```python
from build123d import *

# Parameters (mm, degrees)
BOSS_EXTRUDE1_DEPTH = 11.1125
SKETCH2_R           = 3.5687
CUT_EXTRUDE1_DEPTH  = 51.8
SKETCH3_R           = 3.5687
CUT_EXTRUDE2_DEPTH  = 51.8
CUT_EXTRUDE3_REACH  = 6.775
SKETCH4_W           = 25.4
SKETCH4_H           = 22.225


with BuildPart() as part:
    # Sketch1 → Boss-Extrude1 (new body, symmetric)
    with BuildSketch(Plane.XY):
        with BuildLine():
            Line((0, 0), (0, 50.8))
            ThreePointArc((0, 50.8), (3.376576302, 49.401376302), (4.7752, 46.0248))
            Line((4.7752, 46.0248), (4.7752, 7.9502))
            ThreePointArc((4.7752, 7.9502), (5.70513597, 5.70513597), (7.9502, 4.7752))
            Line((7.9502, 4.7752), (46.0248, 4.7752))
            ThreePointArc((46.0248, 4.7752), (49.401376302, 3.376576302), (50.8, 0))
            Line((50.8, 0), (0, 0))
        make_face()
    extrude(amount=BOSS_EXTRUDE1_DEPTH, both=True)

    # Sketch2 → Cut-Extrude1 (cut, through all)
    with BuildSketch(Plane(origin=(0, 0, 0), x_dir=(1, 0, 0), z_dir=(0, 1, 0))):
        with Locations((12.7, 0)):
            Circle(SKETCH2_R)
        with Locations((38.1, 0)):
            Circle(SKETCH2_R)
    extrude(amount=CUT_EXTRUDE1_DEPTH, mode=Mode.SUBTRACT)

    # Sketch3 → Cut-Extrude2 (cut, through all)
    with BuildSketch(Plane(origin=(0, 0, 0), x_dir=(0, 0, -1), z_dir=(1, 0, 0))):
        with Locations((0, 12.7)):
            Circle(SKETCH3_R)
        with Locations((0, 38.1)):
            Circle(SKETCH3_R)
    extrude(amount=CUT_EXTRUDE2_DEPTH, mode=Mode.SUBTRACT)

    # Sketch4 → Cut-Extrude3 (cut, up to next)
    with BuildSketch(Plane(origin=(0, 4.7752, 0), x_dir=(1, 0, 0), z_dir=(0, 1, 0)), mode=Mode.PRIVATE) as cut_extrude3_sk1:
        with Locations((38.1, 0)):
            Rectangle(SKETCH4_W, SKETCH4_H)
    cut_extrude3_tool1 = extrude(cut_extrude3_sk1.sketch, amount=-CUT_EXTRUDE3_REACH, mode=Mode.PRIVATE) & part.part
    add(cut_extrude3_tool1.solids().sort_by_distance((38.1, 4.7752, 0))[0], mode=Mode.SUBTRACT)


solid = part.part
```
Work out the finished part from the listing and answer in its coordinate system (mm). A direction names the side the tool comes from. Give positions to 0.01 mm unless a question says otherwise; leave off trailing zeros. Order: outer loops, then holes, each group sorted by start corner. A loop starts at its lowest first (then second) coordinate and runs counter-clockwise, first axis right, second up. Notation, with made-up numbers: (48.25, -5) -> (103.25, -5) arc R26 ccw to (103.25, 19) -> close; hole circle Ø1 at (-11.5, 4.5). An arc over 180 degrees is marked (long way). Answer as CSV lines item,"result". Start each with the question number.
(1) Section D-D, the plane z = 5 is taken. Write down the section's boundary in (x, y) (3 decimals).
(2) Which of the six approach directions +Z, -Z, +X, -X, +Y, -Y give full straight-line access (tool end or side, diameter ignored) to faces 4 (the flat face through (4.775, 27, 0)), 5 (the cylindrical face through (9.135, 2.354, -0.157))?
(3) Section A-A, the plane x = 12.7 is taken. Write down the section's boundary in (y, z), plus the area to 3 significant figures.
(4) Consider line 1 along Z through (x, y) = (3.05, 12.7); line 2 along X through (y, z) = (2.5, 0); line 3 along Y through (x, z) = (4.25, 0.25). Determine where each line is inside the solid, lowest interval first.
(5) For a pull along Z with two mould halves and no side action, classify faces 1 (the cylindrical face through (2.354, 9.216, 0.774)), 2 (the flat face through (17, 4.775, 0)), 3 (the flat face through (4, 18, -11.112)) as released by +Z, released by -Z, zero draft, split by the parting line, or undercut.
(6) Section C-C, the plane z = 0 is taken. Write down the section's boundary in (x, y) (3 decimals), plus the area to 3 significant figures.
(7) Each of these flat-tipped pins is pushed along its axis until it touches: pin 1 Ø2 at (y, z) = (19, -6.5) entering from +X; pin 2 Ø9.5 at (x, z) = (12.7, 0) entering from +Y; pin 3 Ø11.5 at (y, z) = (12.7, 0) entering from +X. Where does it stop, or does it pass through?
Entries:
1,outline,"(0, 0) -> (25.4, 0) -> (25.4, 4.775) -> (7.95, 4.775) arc R3.175 cw to (4.775, 7.95) -> (4.775, 46.025) arc R4.775 ccw to (0, 50.8) -> close"
2,face 4,"+Z, -Z, +X, +Y"
2,face 5,"+Y, -Y"
3,outline,"(0, -11.11) -> (4.78, -11.11) -> (4.78, -3.57) -> (0, -3.57) -> close; (0, 3.57) -> (4.78, 3.57) -> (4.78, 11.11) -> (0, 11.11) -> close"
3,area,"72.0 mm²"
4,line 1,"-11.11 to -3.57, 3.57 to 11.11"
4,line 2,"0 to 9.13, 16.27 to 25.4"
4,line 3,"0 to 9.14, 16.26 to 34.54, 41.66 to 48.2"
5,face 1,"undercut"
5,face 2,"zero draft"
5,face 3,"released by -Z"
6,outline,"(0, 0) -> (9.131, 0) -> (9.131, 4.775) -> (7.95, 4.775) arc R3.175 cw to (4.775, 7.95) -> (4.775, 9.131) -> (0, 9.131) -> close; (0, 16.269) -> (4.775, 16.269) -> (4.775, 34.531) -> (0, 34.531) -> close; (0, 41.669) -> (4.775, 41.669) -> (4.775, 46.025) arc R4.775 ccw to (0, 50.8) -> close; (16.269, 0) -> (25.4, 0) -> (25.4, 4.775) -> (16.269, 4.775) -> close"
6,area,"236 mm²"
7,pin 1,"x = 4.78"
7,pin 2,"y = 4.78"
7,pin 3,"x = 4.94"
